```python
from build123d import *

# Parameters (mm, degrees)
F1_DEPTH = 3
F2_W     = 1.5
F2_H     = 70
F3_DEPTH = 1.5


with BuildPart() as f1:
    # F0 (on Front) → F1 (new body)
    with BuildSketch(Plane.XZ):
        Polygon((10, 0), (5, 0), (5, 50), (0, 50), (0, 0), (0, -20), (10, -20), align=None)
    extrude(amount=F1_DEPTH)

    # F2 (on face) → F3 (cut)
    with BuildSketch(Plane.XZ.offset(3)):
        with Locations((2.5, 15)):
            Rectangle(F2_W, F2_H)
    extrude(amount=-F3_DEPTH, mode=Mode.SUBTRACT)


solid = f1.part
```
The listing builds one solid part. Answer for the finished solid, in the listing's coordinates (mm). A direction names the side the tool comes from. Coordinates: 2 decimals unless noted, no trailing zeros. Write each loop counter-clockwise with the first axis right and the second up, starting at its lowest first coordinate (ties: lowest second). Pieces come first, ordered by that corner, then holes. Notation, with made-up numbers: (2, -3.5) - (12, -3.5) arc R13 ccw to (12, 17.5) - close; hole circle Ø1 at (-33.5, 5.5). An arc over 180 degrees is marked (long way). One line per item, written item: value.
1) Consider line 1 along X through (y, z) = (-1.6, 8); line 2 along X through (y, z) = (-2.3, -14.5); line 3 along Y through (x, z) = (3, 11.5). Determine where each line is inside the solid, lowest interval first. Write a range as from..to.
Geometry check:
line 1: x = 0..1.75, 3.25..5
line 2: x = 0..1.75, 3.25..10
line 3: y = -1.5..0
2) Find section A-A (y = -2.4). Give the vertices of the cut face in (x, z), and give its area (3 significant figures).
Geometry check:
outline: (0, -20) - (1.75, -20) - (1.75, 50) - (0, 50) - close; (3.25, -20) - (10, -20) - (10, 0) - (5, 0) - (5, 50) - (3.25, 50) - close
area: 345 mm2
3) Find section C-C (x = 6). Give the vertices of the cut face in (y, z), and give its area (3 significant figures).
Geometry check:
outline: (-3, -20) - (0, -20) - (0, 0) - (-3, 0) - close
area: 60.0 mm2
4) A tool of negligible diameter and unlimited length cuts with its end or side. For faces 1 (the flat face through (3.25, -2, 15)), 2 (the flat face through (8, -1, 0)), 3 (the flat face through (1, -3, 15)), from which of +Z, -Z, +X, -X, +Y, -Y can it reach the whole face along a straight path? Write none if from no direction.
Geometry check:
face 1: +Z, -Z, -Y
face 2: +Z, +X, +Y, -Y
face 3: +Z, -Z, +X, -X, -Y
5) Find section B-B (z = 5.5). Give the vertices of the cut face in (x, y).
Geometry check:
outline: (0, -3) - (1.75, -3) - (1.75, -1.5) - (3.25, -1.5) - (3.25, -3) - (5, -3) - (5, 0) - (0, 0) - close
6) Find section D-D (z = -11). Give the vertices of the cut face in (x, y), and give its area (4 significant figures).
Geometry check:
outline: (0, -3) - (1.75, -3) - (1.75, -1.5) - (3.25, -1.5) - (3.25, -3) - (10, -3) - (10, 0) - (0, 0) - close
area: 27.75 mm2
7) For a pull along X with two mould halves and no side action, classify faces 4 (the flat face through (1.75, -2, 15)), 5 (the flat face through (5, -1, 25)), 6 (the flat face through (4, -3, 0)), 7 (the flat face through (0, -1, 15)) as pulls with the +X half, pulls with the -X half, needs draft (parallel to the pull), parting line crosses it, or undercut.
Geometry check:
face 4: undercut
face 5: pulls with the +X half
face 6: needs draft
face 7: pulls with the -X half
8) Each of these flat-tipped pins is pushed along its axis until it touches: pin 1 Ø0.9 at (y, z) = (-2, 26.5) entering from +X; pin 2 Ø1.2 at (x, z) = (2.5, -1.5) entering from -Y. Where does it stop, or does it pass through?
Geometry check:
pin 1: stops at x = 5
pin 2: stops at y = -1.5
